Study the drawing (mm; zero at the part's minimum x, y, z) and answer. A direction names the side the tool comes from. Round coordinates to 2 decimals unless told otherwise and drop trailing zeros. Order: outer loops, then holes, each group sorted by start corner. A loop starts at its lowest first (then second) coordinate and runs counter-clockwise, first axis right, second up. Notation, with made-up numbers: (-24.75, -10.75) -> (-0.75, -10.75) arc R23 cw to (-0.75, 2.25) -> close; hole circle Ø1 at (76.5, 68.5). An arc over 180 degrees is marked (long way). Use one line per item in the form item = value.
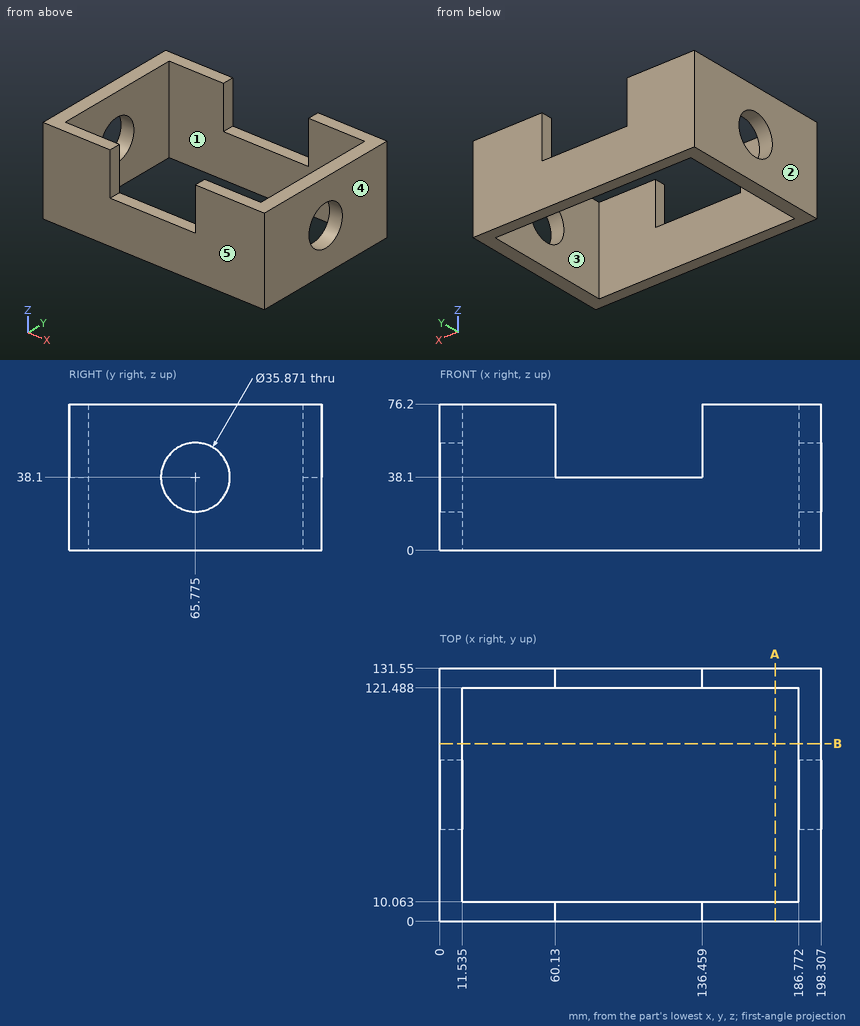
Item 1: For the marked faces 1 and 2, determine the directions among +Z, -Z, +X, -X, +Y, -Y from which every point of the face is accessible in a straight line to the end or side of a thin tool.
Findings:
face_1 = +Z, -Z
face_2 = +Z, -Z, -X, +Y, -Y
Item 2: A flat-ended cylindrical pin translates along its axis: P1, Ø8, axis at x = 100, y = 7, coming from the +Z side. Find the tip coordinate at first contact, or state that the pin passes through.
Findings:
P1 = 38.1
Item 3: The part is cut by section B-B, the plane y = 92.5. Give the vertices of the cut face in (x, z) (1 decimal), and give its area (3 significant figures).
Findings:
outline = (0, 0) -> (11.5, 0) -> (11.5, 76.2) -> (0, 76.2) -> close; (186.8, 0) -> (198.3, 0) -> (198.3, 76.2) -> (186.8, 76.2) -> close
area = 1,760 mm^2
Item 4: The part is cut by section A-A, the plane x = 174.5. Give the vertices of the cut face in (y, z), and give its area (3 significant figures).
Findings:
outline = (0, 0) -> (10.06, 0) -> (10.06, 76.2) -> (0, 76.2) -> close; (121.49, 0) -> (131.55, 0) -> (131.55, 76.2) -> (121.49, 76.2) -> close
area = 1,530 mm^2
Item 5: Consider line 1 along Y through (x, z) = (45.5, 5); line 2 along X through (y, z) = (26.5, 22) (1 decimal). Determine where each line is inside the solid, lowest interval first.
Findings:
line_1 = 0 to 10.06, 121.49 to 131.55
line_2 = 0 to 11.5, 186.8 to 198.3
Item 6: Determine the mould class of the marked faces 3, 4 and 5 for opening direction Y: released by +Y, released by -Y, zero draft, split by the parting line, or undercut.
Findings:
face_3 = undercut
face_4 = zero draft
face_5 = released by -Y
